Can you work these out from the model? Positions are in its coordinate system, mm. A direction names the side the tool comes from. Give positions to 0.01 mm unless a question says otherwise; leave off trailing zeros. Write each loop counter-clockwise with the first axis right and the second up, starting at its lowest first coordinate (ties: lowest second). Pieces come first, ordered by that corner, then holes. Notation, with made-up numbers: (10.25, 20.5) -> (47.25, 20.5) arc R35 cw to (47.25, 56.5) -> close; hole circle Ø11 at (31, 78). An arc over 180 degrees is marked (long way). Answer as CSV lines item,"result". Start each with the question number.
1. If we section it at B-B on x = -98: Write out the boundary of the cut face in (y, z), plus the area to 3 significant figures.
2. If we section it at A-A on z = 10.5: Write out the boundary of the cut face in (x, y), plus the area to 3 significant figures.
3. I'm going to push a flat-ended pin straight in: P1, Ø1.5, axis at x = 30, y = 131, coming from the -Z side. Where does the tip first touch, or does it pass through?
4. I need wall thicknesses on line 1 (Y direction, x = -121.5, z = 18); line 2 (X direction, y = -552, z = 9.5); line 3 (Y direction, x = 405, z = 2.75). Which ranges of each line are inside material? Lowest first, please. Write a range as [from, to].
5. If we section it at C-C on y = -279: Write out the boundary of the cut face in (x, z).
6. If we mould it in two halves opening along X, with no side actions, what happens to faces 3 (the face through (8, 12, 27)), 4 (the face through (-8, 12, 30))? For each: pulls with the +X half, pulls with the -X half, needs draft (parallel to the pull), parting line crosses it, or undercut.
7. On a 3-axis mill with a long thin cutter (end or side, diameter ignored), from which of +Z, -Z, +X, -X, +Y, -Y can I reach the whole of each face in a straight line? I mean faces 1 (the face through (545, 4, 3)), 2 (the face through (-549, 4, 0)). Say none if no direction works.
```python
from build123d import *

# Parameters (mm, degrees)
ESQUISSE1_W             = 1134
ESQUISSE1_H             = 1722
BOSS_EXTRU_1_DEPTH      = 30
ESQUISSE6_W             = 1038.990735542
ESQUISSE6_H             = 1577.726672488
ENL_V_MAT_EXTRU_1_DEPTH = 27
ESQUISSE7_W             = 1127.272234852
ESQUISSE7_H             = 1708.57841833
ENL_V_MAT_EXTRU_2_DEPTH = 24
ENL_V_MAT_EXTRU_3_DEPTH = 10


with BuildPart() as part:
    # Esquisse1 → Boss.-Extru.1 (new body)
    with BuildSketch(Plane.XY):
        Rectangle(ESQUISSE1_W, ESQUISSE1_H)
    extrude(amount=BOSS_EXTRU_1_DEPTH)

    # Esquisse6 → Enlèv. mat.-Extru.1 (cut)
    with BuildSketch(Plane(origin=(0, 0, 0), x_dir=(-1, 0, 0), z_dir=(0, 0, -1))):
        Rectangle(ESQUISSE6_W, ESQUISSE6_H)
    extrude(amount=-ENL_V_MAT_EXTRU_1_DEPTH, mode=Mode.SUBTRACT)

    # Esquisse7 → Enlèv. mat.-Extru.2 (cut)
    with BuildSketch(Plane(origin=(0, 0, 27), x_dir=(-1, 0, 0), z_dir=(0, 0, -1))):
        Rectangle(ESQUISSE7_W, ESQUISSE7_H)
    extrude(amount=ENL_V_MAT_EXTRU_2_DEPTH, mode=Mode.SUBTRACT)

    # trous fixation → Enlèv. mat.-Extru.3 (cut)
    with BuildSketch(Plane(origin=(0, 0, 0), x_dir=(-1, 0, 0), z_dir=(0, 0, -1))):
        with BuildLine():
            Line((-543.5, 693), (-542.5, 693))
            ThreePointArc((-542.5, 693), (-539.671572875, 694.171572875), (-538.5, 697))
            Line((-538.5, 697), (-538.5, 703))
            ThreePointArc((-538.5, 703), (-539.671572875, 705.828427125), (-542.5, 707))
            Line((-542.5, 707), (-543.5, 707))
            ThreePointArc((-543.5, 707), (-546.328427125, 705.828427125), (-547.5, 703))
            Line((-547.5, 703), (-547.5, 697))
            ThreePointArc((-547.5, 697), (-546.328427125, 694.171572875), (-543.5, 693))
        make_face()
        with BuildLine():
            Line((-543.5, 423), (-542.5, 423))
            ThreePointArc((-542.5, 423), (-539.671572875, 424.171572875), (-538.5, 427))
            Line((-538.5, 427), (-538.5, 433))
            ThreePointArc((-538.5, 433), (-539.671572875, 435.828427125), (-542.5, 437))
            Line((-542.5, 437), (-543.5, 437))
            ThreePointArc((-543.5, 437), (-546.328427125, 435.828427125), (-547.5, 433))
            Line((-547.5, 433), (-547.5, 427))
            ThreePointArc((-547.5, 427), (-546.328427125, 424.171572875), (-543.5, 423))
        make_face()
        with BuildLine():
            Line((-543.5, -437), (-542.5, -437))
            ThreePointArc((-542.5, -437), (-539.671572875, -435.828427125), (-538.5, -433))
            Line((-538.5, -433), (-538.5, -427))
            ThreePointArc((-538.5, -427), (-539.671572875, -424.171572875), (-542.5, -423))
            Line((-542.5, -423), (-543.5, -423))
            ThreePointArc((-543.5, -423), (-546.328427125, -424.171572875), (-547.5, -427))
            Line((-547.5, -427), (-547.5, -433))
            ThreePointArc((-547.5, -433), (-546.328427125, -435.828427125), (-543.5, -437))
        make_face()
        with BuildLine():
            Line((-543.5, -707), (-542.5, -707))
            ThreePointArc((-542.5, -707), (-539.671572875, -705.828427125), (-538.5, -703))
            Line((-538.5, -703), (-538.5, -697))
            ThreePointArc((-538.5, -697), (-539.671572875, -694.171572875), (-542.5, -693))
            Line((-542.5, -693), (-543.5, -693))
            ThreePointArc((-543.5, -693), (-546.328427125, -694.171572875), (-547.5, -697))
            Line((-547.5, -697), (-547.5, -703))
            ThreePointArc((-547.5, -703), (-546.328427125, -705.828427125), (-543.5, -707))
        make_face()
        with BuildLine():
            Line((538.5, -703), (538.5, -697))
            ThreePointArc((538.5, -697), (539.671572875, -694.171572875), (542.5, -693))
            Line((542.5, -693), (543.5, -693))
            ThreePointArc((543.5, -693), (546.328427125, -694.171572875), (547.5, -697))
            Line((547.5, -697), (547.5, -703))
            ThreePointArc((547.5, -703), (546.328427125, -705.828427125), (543.5, -707))
            Line((543.5, -707), (542.5, -707))
            ThreePointArc((542.5, -707), (539.671572875, -705.828427125), (538.5, -703))
        make_face()
        with BuildLine():
            Line((538.5, -433), (538.5, -427))
            ThreePointArc((538.5, -427), (539.671572875, -424.171572875), (542.5, -423))
            Line((542.5, -423), (543.5, -423))
            ThreePointArc((543.5, -423), (546.328427125, -424.171572875), (547.5, -427))
            Line((547.5, -427), (547.5, -433))
            ThreePointArc((547.5, -433), (546.328427125, -435.828427125), (543.5, -437))
            Line((543.5, -437), (542.5, -437))
            ThreePointArc((542.5, -437), (539.671572875, -435.828427125), (538.5, -433))
        make_face()
        with BuildLine():
            Line((538.5, 427), (538.5, 433))
            ThreePointArc((538.5, 433), (539.671572875, 435.828427125), (542.5, 437))
            Line((542.5, 437), (543.5, 437))
            ThreePointArc((543.5, 437), (546.328427125, 435.828427125), (547.5, 433))
            Line((547.5, 433), (547.5, 427))
            ThreePointArc((547.5, 427), (546.328427125, 424.171572875), (543.5, 423))
            Line((543.5, 423), (542.5, 423))
            ThreePointArc((542.5, 423), (539.671572875, 424.171572875), (538.5, 427))
        make_face()
        with BuildLine():
            Line((538.5, 697), (538.5, 703))
            ThreePointArc((538.5, 703), (539.671572875, 705.828427125), (542.5, 707))
            Line((542.5, 707), (543.5, 707))
            ThreePointArc((543.5, 707), (546.328427125, 705.828427125), (547.5, 703))
            Line((547.5, 703), (547.5, 697))
            ThreePointArc((547.5, 697), (546.328427125, 694.171572875), (543.5, 693))
            Line((543.5, 693), (542.5, 693))
            ThreePointArc((542.5, 693), (539.671572875, 694.171572875), (538.5, 697))
        make_face()
    extrude(amount=-ENL_V_MAT_EXTRU_3_DEPTH, mode=Mode.SUBTRACT)


solid = part.part
```
Computed values:
1,outline,"(-861, 0) -> (-788.86, 0) -> (-788.86, 3) -> (-854.29, 3) -> (-854.29, 27) -> (854.29, 27) -> (854.29, 3) -> (788.86, 3) -> (788.86, 0) -> (861, 0) -> (861, 30) -> (-861, 30) -> close"
1,area,"5,920 mm2"
2,outline,"(-567, -861) -> (567, -861) -> (567, 861) -> (-567, 861) -> close; hole (-563.64, -854.29) -> (563.64, -854.29) -> (563.64, 854.29) -> (-563.64, 854.29) -> close"
2,area,"26,700 mm2"
3,P1,"stops at z = 27"
4,line 1,"y = [-861, -854.29], [854.29, 861]"
4,line 2,"x = [-567, -563.64], [563.64, 567]"
4,line 3,"y = [-861, -788.86], [788.86, 861]"
5,outline,"(-567, 0) -> (-519.5, 0) -> (-519.5, 3) -> (-563.64, 3) -> (-563.64, 27) -> (563.64, 27) -> (563.64, 3) -> (519.5, 3) -> (519.5, 0) -> (567, 0) -> (567, 30) -> (-567, 30) -> close"
6,face 3,"undercut"
6,face 4,"needs draft"
7,face 1,"none"
7,face 2,"-Z, +X, -X, +Y, -Y"
